Check sheet for the drawn part. Datum: minimum x, y, z corner. Units: mm. A direction names the side the tool comes from. Give positions to 0.01 mm unless a question says otherwise; leave off trailing zeros. Write each loop counter-clockwise with the first axis right and the second up, starting at its lowest first coordinate (ties: lowest second). Pieces come first, ordered by that corner, then holes. Notation, with made-up numbers: (68, 40) - (98, 40) arc R23 ccw to (98, 58) - close; hole circle Ø6 at (22.5, 78.5). An arc over 180 degrees is marked (long way). Answer as a JSON object with one key per item and string values. Group by question number.
Item 1: Sectioned sample at D-D, the plane x = 57.15. Record the boundary of the cut face in (y, z) (3 decimals), and give its area (3 significant figures).
Item 2: Sectioned sample at C-C, the plane x = 31.75. Record the boundary of the cut face in (y, z) (3 decimals), and give its area (3 significant figures).
Item 3: Draft check along Z on the marked faces 1, 2, 3 and 4. Enter one of: +Z half, -Z half, draft (parallel to the pull), parting line (faces both ways), or undercut.
Item 4: Scan lines: line 1 along Z through (x, y) = (31.75, 18.75); line 2 along X through (y, z) = (15, 65); line 3 along Z through (x, y) = (61.5, 18.25). Record each from-to range of solid material in increasing order. Write a range as [from, to].
Item 5: Tool access check on the marked faces 5, 6 and 7. Record the directions out of +Z, -Z, +X, -X, +Y, -Y that give a thin tool (end or side, any length) a straight path to the whole face; none if there is none.
Item 6: Sectioned sample at A-A, the plane z = 44.45. Record the boundary of the cut face in (x, y) (3 decimals), and give its area (3 significant figures).
Item 7: Go/stop test with flat-tipped pins: pin 1 (8.5 mm diameter, centred on y = 9.5, z = 53.5, fed in from +X); pin 2 (5 mm diameter, centred on x = 57.5, z = 59.5, fed in from -Y); pin 3 (12.5 mm diameter, centred on x = 11.5, y = 13, fed in from +Z); pin 4 (4 mm diameter, centred on x = 82.5, y = 13, fed in from +Z). Record where each tip stops, or that it passes through.
Item 8: Sectioned sample at B-B, the plane y = 17. Record the boundary of the cut face in (x, z).
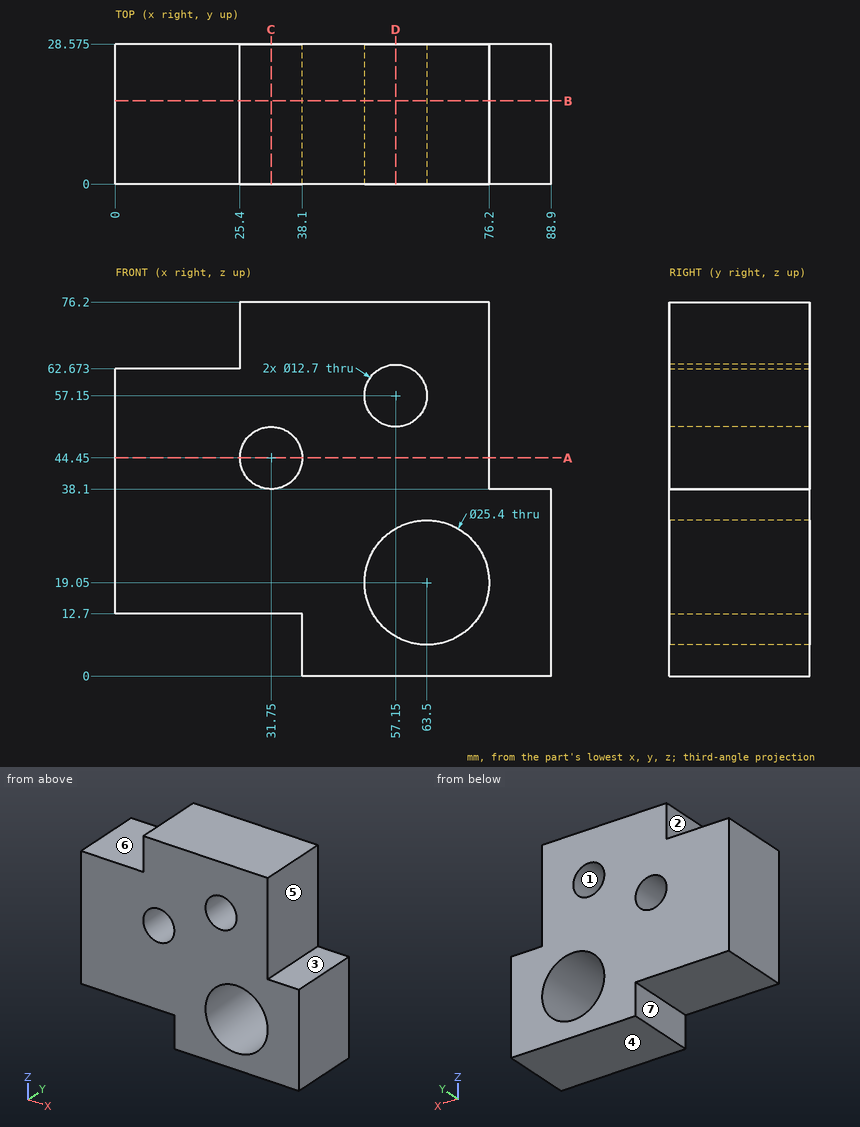
Geometry check:
{
 "1": {"outline": "(0, 0) - (28.575, 0) - (28.575, 8.051) - (0, 8.051) - close; (0, 30.049) - (28.575, 30.049) - (28.575, 50.8) - (0, 50.8) - close; (0, 63.5) - (28.575, 63.5) - (28.575, 76.2) - (0, 76.2) - close", "area": "1,190 mm^2"},
 "2": {"outline": "(0, 12.7) - (28.575, 12.7) - (28.575, 38.1) - (0, 38.1) - close; (0, 50.8) - (28.575, 50.8) - (28.575, 76.2) - (0, 76.2) - close", "area": "1,450 mm^2"},
 "3": {"face 1": "undercut", "face 2": "draft", "face 3": "+Z half", "face 4": "-Z half"},
 "4": {"line 1": "[12.7, 38.1], [50.8, 76.2]", "line 2": "[25.4, 76.2]", "line 3": "[0, 6.51], [31.59, 52.52], [61.78, 76.2]"},
 "5": {"face 5": "+Z, +X, +Y, -Y", "face 6": "+Z, -X, +Y, -Y", "face 7": "-Z, -X, +Y, -Y"},
 "6": {"outline": "(0, 0) - (25.4, 0) - (25.4, 28.575) - (0, 28.575) - close; (38.1, 0) - (76.2, 0) - (76.2, 28.575) - (38.1, 28.575) - close", "area": "1,810 mm^2"},
 "7": {"pin 1": "x = 76.2", "pin 2": "through", "pin 3": "z = 62.67", "pin 4": "z = 38.1"},
 "8": {"outline": "(0, 12.7) - (38.1, 12.7) - (38.1, 0) - (88.9, 0) - (88.9, 38.1) - (76.2, 38.1) - (76.2, 76.2) - (25.4, 76.2) - (25.4, 62.67) - (0, 62.67) - close; hole circle Ø12.7 at (31.75, 44.45); hole circle Ø25.4 at (63.5, 19.05); hole circle Ø12.7 at (57.15, 57.15)"}
}
